Check sheet for the modelled part. Datum: model origin and axes. Units: mm. Face numbers are marked on the shaded views. Give positions to 0.01 mm unless a question says otherwise; leave off trailing zeros. Order: outer loops, then holes, each group sorted by start corner. A loop starts at its lowest first (then second) coordinate and runs counter-clockwise, first axis right, second up. Notation, with made-up numbers: (-11.75, 62.25) - (11.25, 62.25) arc R33 cw to (11.25, 97.25) - close; hole circle Ø1 at (66, -38.5). An arc over 180 degrees is marked (long way). Answer in a Markdown table with one row per item.
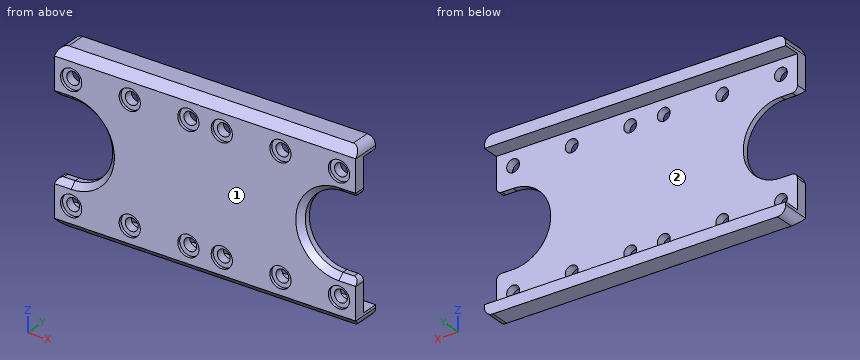
from build123d import *

# Parameters (mm, degrees)
EXTRUDE_1_DEPTH              = 27
CUT_EXTRUDE_1_REACH          = 33.032
HOLE_WIZARD_M2_1_D           = 2.3
HOLE_WIZARD_M2_1_CBORE_D     = 3.8
HOLE_WIZARD_M2_1_CBORE_DEPTH = 0.5
PATTERN_LINEAR_1_COUNT       = 3
PATTERN_LINEAR_1_PITCH       = 10.5
MIRROR_1_COPY_1_D            = 2.3
MIRROR_1_COPY_1_CBORE_D      = 3.8
MIRROR_1_COPY_1_CBORE_DEPTH  = 0.5
MIRROR_1_COPY_2_D            = 2.3
MIRROR_1_COPY_2_CBORE_D      = 3.8
MIRROR_1_COPY_2_CBORE_DEPTH  = 0.5
CHAMFER_1_SIZE               = 1
MIRROR_3_COPY_1_D            = 2.3
MIRROR_3_COPY_1_CBORE_D      = 3.8
MIRROR_3_COPY_1_CBORE_DEPTH  = 0.5
MIRROR_3_COPY_2_D            = 2.3
MIRROR_3_COPY_2_CBORE_D      = 3.8
MIRROR_3_COPY_2_CBORE_DEPTH  = 0.5
MIRROR_3_COPY_3_D            = 2.3
MIRROR_3_COPY_3_CBORE_D      = 3.8
MIRROR_3_COPY_3_CBORE_DEPTH  = 0.5
MIRROR_3_COPY_4_D            = 2.3
MIRROR_3_COPY_4_CBORE_D      = 3.8
MIRROR_3_COPY_4_CBORE_DEPTH  = 0.5
MIRROR_3_COPY_5_D            = 2.3
MIRROR_3_COPY_5_CBORE_D      = 3.8
MIRROR_3_COPY_5_CBORE_DEPTH  = 0.5
CHAMFER_1_OF_MIRROR_3_SIZE   = 1
FILLET_1_R                   = 1.5
FILLET_2_R                   = 1
CHAMFER_2_SIZE               = 1.5


with BuildPart() as part:
    # ｽｹｯﾁ1 → ﾎﾞｽ - 押し出し1 (new, symmetric)
    with BuildSketch(Plane(origin=(0, 0, 0), x_dir=(0, 0, -1), z_dir=(1, 0, 0))):
        Polygon((-15, 0), (15, 0), (15, 5), (13, 5), (13, 2), (-13, 2), (-13, 5), (-15, 5), align=None)
    extrude(amount=EXTRUDE_1_DEPTH, both=True)

    # ｽｹｯﾁ2 → ｶｯﾄ - 押し出し1 (cut, up to next)
    with BuildSketch(Plane(origin=(0, 2, 0), x_dir=(1, 0, 0), z_dir=(0, 1, 0)), mode=Mode.PRIVATE) as cut_extrude_1_sk1:
        with BuildLine():
            Line((24, 6.75), (28, 6.75))
            Line((28, 6.75), (28, -6.75))
            Line((28, -6.75), (24, -6.75))
            ThreePointArc((24, -6.75), (17.25, 0), (24, 6.75))
        make_face()
    cut_extrude_1_tool1 = extrude(cut_extrude_1_sk1.sketch, amount=-CUT_EXTRUDE_1_REACH, mode=Mode.PRIVATE) & part.part
    cut_extrude_1 = cut_extrude_1_tool1.solids().sort_by_distance((23.22727, 2, 0))[0]
    add(cut_extrude_1, mode=Mode.SUBTRACT)

    # M2 丸平ねじ用座ぐり穴1 (through all)
    with Locations(Plane(origin=(0, 0, 0), x_dir=(-1, 0, 0), z_dir=(0, -1, 0))):
        with Locations((-24, -10.5)):
            hole_wizard_m2_1 = CounterBoreHole(HOLE_WIZARD_M2_1_D / 2, HOLE_WIZARD_M2_1_CBORE_D / 2, HOLE_WIZARD_M2_1_CBORE_DEPTH)

    # 直線ﾊﾟﾀｰﾝ1: M2 丸平ねじ用座ぐり穴1 ×3
    with Locations(*[(-i * PATTERN_LINEAR_1_PITCH, 0, 0) for i in range(1, PATTERN_LINEAR_1_COUNT)]):
        add(hole_wizard_m2_1, mode=Mode.SUBTRACT)

    # ﾐﾗｰ1: M2 丸平ねじ用座ぐり穴1 across plane
    add(hole_wizard_m2_1.mirror(Plane.XY), mode=Mode.SUBTRACT)

    # ﾐﾗｰ1 copy 1 (through all)
    with Locations(Plane(origin=(-10.5, 0, 0), x_dir=(-1, 0, 0), z_dir=(0, -1, 0))):
        with Locations((-24, 10.5)):
            CounterBoreHole(MIRROR_1_COPY_1_D / 2, MIRROR_1_COPY_1_CBORE_D / 2, MIRROR_1_COPY_1_CBORE_DEPTH)

    # ﾐﾗｰ1 copy 2 (through all)
    with Locations(Plane(origin=(-21, 0, 0), x_dir=(-1, 0, 0), z_dir=(0, -1, 0))):
        with Locations((-24, 10.5)):
            CounterBoreHole(MIRROR_1_COPY_2_D / 2, MIRROR_1_COPY_2_CBORE_D / 2, MIRROR_1_COPY_2_CBORE_DEPTH)

    # 面取り1
    chamfer_1_edges = [part.edges().sort_by_distance(p)[0] for p in [
        (25.5, 0, 6.75),
        (17.25, 0, 0),
        (25.5, 0, -6.75),
    ]]
    chamfer(chamfer_1_edges, length=CHAMFER_1_SIZE)

    # ﾐﾗｰ3: ｶｯﾄ - 押し出し1, M2 丸平ねじ用座ぐり穴1 across plane
    add(cut_extrude_1.mirror(Plane(origin=(0, 0, 0), x_dir=(0, 0, 1), z_dir=(1, 0, 0))), mode=Mode.SUBTRACT)
    add(hole_wizard_m2_1.mirror(Plane(origin=(0, 0, 0), x_dir=(0, 0, 1), z_dir=(1, 0, 0))), mode=Mode.SUBTRACT)

    # ﾐﾗｰ3 copy 1 (through all)
    with Locations(Plane(origin=(10.5, 0, 0), x_dir=(1, 0, 0), z_dir=(0, -1, 0))):
        with Locations((-24, 10.5)):
            CounterBoreHole(MIRROR_3_COPY_1_D / 2, MIRROR_3_COPY_1_CBORE_D / 2, MIRROR_3_COPY_1_CBORE_DEPTH)

    # ﾐﾗｰ3 copy 2 (through all)
    with Locations(Plane(origin=(21, 0, 0), x_dir=(1, 0, 0), z_dir=(0, -1, 0))):
        with Locations((-24, 10.5)):
            CounterBoreHole(MIRROR_3_COPY_2_D / 2, MIRROR_3_COPY_2_CBORE_D / 2, MIRROR_3_COPY_2_CBORE_DEPTH)

    # ﾐﾗｰ3 copy 3 (through all)
    with Locations(Plane.XZ):
        with Locations((-24, -10.5)):
            CounterBoreHole(MIRROR_3_COPY_3_D / 2, MIRROR_3_COPY_3_CBORE_D / 2, MIRROR_3_COPY_3_CBORE_DEPTH)

    # ﾐﾗｰ3 copy 4 (through all)
    with Locations(Plane(origin=(10.5, 0, 0), x_dir=(1, 0, 0), z_dir=(0, -1, 0))):
        with Locations((-24, -10.5)):
            CounterBoreHole(MIRROR_3_COPY_4_D / 2, MIRROR_3_COPY_4_CBORE_D / 2, MIRROR_3_COPY_4_CBORE_DEPTH)

    # ﾐﾗｰ3 copy 5 (through all)
    with Locations(Plane(origin=(21, 0, 0), x_dir=(1, 0, 0), z_dir=(0, -1, 0))):
        with Locations((-24, -10.5)):
            CounterBoreHole(MIRROR_3_COPY_5_D / 2, MIRROR_3_COPY_5_CBORE_D / 2, MIRROR_3_COPY_5_CBORE_DEPTH)

    # 面取り1 of ﾐﾗｰ3
    chamfer_1_of_mirror_3_edges = [part.edges().sort_by_distance(p)[0] for p in [
        (-25.5, 0, 6.75),
        (-17.25, 0, 0),
        (-25.5, 0, -6.75),
    ]]
    chamfer(chamfer_1_of_mirror_3_edges, length=CHAMFER_1_OF_MIRROR_3_SIZE)

    # ﾌｨﾚｯﾄ1
    fillet_1_edges = [part.edges().sort_by_distance(p)[0] for p in [
        (27, 2.5, -15),
        (-27, 2.5, 15),
        (27, 2.5, 15),
        (-27, 2.5, -15),
    ]]
    fillet(fillet_1_edges, radius=FILLET_1_R)

    # ﾌｨﾚｯﾄ2
    fillet_2_edges = [part.edges().sort_by_distance(p)[0] for p in [
        (27, 1.5, -6.75),
        (27, 1.5, 6.75),
        (-27, 1.5, -6.75),
        (-27, 1.5, 6.75),
    ]]
    fillet(fillet_2_edges, radius=FILLET_2_R)

    # 面取り2
    # the kernel refuses this chamfer: 1.5 mm, written as the material it takes off along each edge
    with BuildSketch(Plane(origin=(-29.357524482, 0, -15), x_dir=(0, -0.027495876610586542, 0.9996219169112968), z_dir=(1, 0, 0)), Plane(origin=(29.357524482, 0, 15), x_dir=(0, -0.027495876610586178, -0.9996219169112968), z_dir=(-1, 0, 0))) as chamfer_2_piece_1:
        Polygon((CHAMFER_2_SIZE * 0.999621916911, -CHAMFER_2_SIZE * 0.0274958766106), (-CHAMFER_2_SIZE * 0.0274958766106, -CHAMFER_2_SIZE * 0.999621916911), (0, 0), align=None)
    extrude(amount=58.715048964, mode=Mode.SUBTRACT)


solid = part.part
(1) Cross-section at C-C, the plane x = 10. Record the cut outline in (y, z).
Geometry says:
| item | result |
|---|---|
| outline | (0, -13.5) - (1.5, -15) - (5, -15) - (5, -13) - (2, -13) - (2, 13) - (5, 13) - (5, 15) - (1.5, 15) - (0, 13.5) - close |
(2) Thickness scan on L1, parallel to Z at x = 9, y = 3.95; L2, parallel to Z at x = -3, y = 0.2; L3, parallel to Z at x = 4, y = 1.9. Record the ranges inside material, lowest first.
Geometry says:
| item | result |
|---|---|
| L1 | -15 to -13, 13 to 15 |
| L2 | -13.7 to -12.4, -8.6 to 8.6, 12.4 to 13.7 |
| L3 | -15 to -11.07, -9.93 to 9.93, 11.07 to 15 |
(3) Cross-section at D-D, the plane z = 10.5. Give the number of separate pieces and of enclosed holes in the cut face, then the cut area to 3 significant figures.
Geometry says:
| item | result |
|---|---|
| separate pieces | 7 |
| enclosed holes | 0 |
| area | 75.9 mm² |
(4) Mould release check, pull along Z, two halves, no side actions. Record for the marked faces 1 and 2: pulls with the +Z half, pulls with the -Z half, needs draft (parallel to the pull), parting line crosses it, or undercut.
Geometry says:
| item | result |
|---|---|
| face 1 | needs draft |
| face 2 | undercut |
(5) Cross-section at B-B, the plane y = 4.4. Record the cut outline in (x, z).
Geometry says:
| item | result |
|---|---|
| outline | (-27, -13.5) arc R1.5 ccw to (-25.5, -15) - (25.5, -15) arc R1.5 ccw to (27, -13.5) - (27, -13) - (-27, -13) - close; (-27, 13) - (27, 13) - (27, 13.5) arc R1.5 ccw to (25.5, 15) - (-25.5, 15) arc R1.5 ccw to (-27, 13.5) - close |
(6) Gauge pin test, flat ends, axial feed: P1, Ø1.5, axis at x = 12, y = 0.5, coming from the -Z side; P2, Ø3.5, axis at x = 13.5, z = -10.5, coming from the -Y side. Record the tip position at first contact, or that the pin passes through.
Geometry says:
| item | result |
|---|---|
| P1 | z = -14.75 |
| P2 | y = 0.5 |
(7) Cross-section at A-A, the plane x = -3. Record the cut outline in (y, z), then the cut area to 4 significant figures.
Geometry says:
| item | result |
|---|---|
| outline | (0, -13.5) - (1.5, -15) - (5, -15) - (5, -13) - (2, -13) - (2, -11.65) - (0.5, -11.65) - (0.5, -12.4) - (0, -12.4) - close; (0, -8.6) - (0.5, -8.6) - (0.5, -9.35) - (2, -9.35) - (2, 9.35) - (0.5, 9.35) - (0.5, 8.6) - (0, 8.6) - close; (0, 12.4) - (0.5, 12.4) - (0.5, 11.65) - (2, 11.65) - (2, 13) - (5, 13) - (5, 15) - (1.5, 15) - (0, 13.5) - close |
| area | 59.05 mm² |
